Autodesk Inventor part; units mm, degrees
ref_plane "YZ Plane" through (0, 0, 0) normal (1, 0, 0) x (0, 1, 0)
ref_plane "XZ Plane" through (0, 0, 0) normal (0, 1, 0) x (-1, 0, 0)
ref_plane "XY Plane" through (0, 0, 0) normal (0, 0, 1) x (1, 0, 0)
sketch "Sketch1" plane through (0, 0, 0) normal (0, 1, 0) x (-1, 0, 0)
  line L0 (-9.2054, 64.0966) -> (-85.4054, 64.0966)
  line L1 (-85.4054, 64.0966) -> (-85.4054, -88.3034)
  line L2 (-85.4054, -88.3034) -> (-9.2054, -88.3034)
  line L3 (-9.2054, -88.3034) -> (-9.2054, 64.0966)
  point P0 (0, 0)
  dimension "d0" = 152.4
  dimension "d1" = 76.2
extrude "Plate1" add sketch "Sketch1" along normal blind 3.048
sketch "Sketch2" plane through (82.3574, 0, -88.3034) normal (1, 0, 0) x (0, 1, 0)
  line L0 (0, 152.4) -> (0, 0)
  line L1 (0, 0) -> (152.4, 0)
  line L2 (152.4, 0) -> (152.4, 152.4)
  line L3 (152.4, 152.4) -> (0, 152.4)
edge flange "Flange1" height 152.4 angle 90 thickness 3.048 bend radius 3.048 thickness toward (1, 0, 0) relief tear relief width 3.048 relief depth 1.524 edges at (85.4054, 3.048, -12.1034) wall of the first edge with corners at (82.3574, 0, 64.0966) (82.3574, 0, -88.3034) (82.3574, 152.4, -88.3034) (82.3574, 152.4, 64.0966)
bend "Bend1"
corner "Corner1"
sketch "Sketch3" plane through (85.4054, 152.4, 64.0966) normal (1, 0, 0) x (0, 0, -1)
  circle A0 centre (57.15, -76.2) radius 38.1
  line L0 (152.4, 0) -> (152.4, -146.304)
  line L1 (152.4, -152.4) -> (0, -152.4)
  point P0 (64.0966, -152.4)
  dimension "d13" = 76.2
  dimension "d14" = 95.25
  dimension "d15" = 76.2
extrude "Cut1" cut sketch "Sketch3" against normal blind 3.048
sketch "Sketch4" plane through (85.4054, 152.4, 64.0966) normal (1, 0, 0) x (0, 0, -1)
  circle A0 centre (57.15, -76.2) radius 38.1
  line L0 (19.05, -76.2) -> (19.05, 0)
  line L1 (19.05, 0) -> (31.75, 0)
  line L2 (0, 0) -> (152.4, 0)
  line L3 (19.05, 0) -> (31.75, 0)
  line L4 (31.75, 0) -> (31.75, -47.8019)
  arc A1 (31.75, -47.8019) -> (19.05, -76.2) centre (57.15, -76.2) ccw
  point P0 (64.0966, -152.4)
  dimension "d18" = 12.7
extrude "Cut2" cut sketch "Sketch4" against normal blind 3.048 contours A0 L0 L1 L4
sketch "Sketch5" plane through (82.3574, 149.352, 32.3466) normal (0, 1, 0) x (-1, 0, 0)
  line L0 (0, -120.65) -> (0, 0)
  line L1 (0, 0) -> (-114.3, 0)
  line L2 (-114.3, 0) -> (-114.3, -120.65)
  line L3 (-114.3, -120.65) -> (0, -120.65)
edge flange "Flange2" height 114.3 angle 90 thickness 3.048 bend radius 3.048 thickness toward (0, 1, 0) relief tear relief width 3.048 relief depth 1.524 edges at (85.4054, 152.4, -27.9784) wall of the first edge with corners at (82.3574, 149.352, -88.3034) (82.3574, 149.352, 32.3466) (196.6574, 149.352, 32.3466) (196.6574, 149.352, -88.3034)
bend "Bend2"
corner "Corner2"
sketch "Sketch6" plane through (196.6574, 152.4, 32.3466) normal (0, 1, 0) x (1, 0, 0)
  line L0 (0, 120.65) -> (0, 0)
  line L1 (0, 0) -> (-108.204, 0)
  point P0 (-196.6574, 32.3466)
sketch "Sketch7" plane through (82.3574, 149.352, 64.0966) normal (0, 1, 0) x (-1, 0, 0)
  line L0 (0, -19.05) -> (0, 0)
  line L1 (0, 0) -> (-44.45, 0)
  line L2 (-44.45, 0) -> (-44.45, -19.05)
  line L3 (-44.45, -19.05) -> (0, -19.05)
edge flange "Flange3" height 44.45 angle 90 thickness 3.048 bend radius 3.048 thickness toward (0, 1, 0) relief tear relief width 3.048 relief depth 1.524 edges at (85.4054, 152.4, 54.5716) wall of the first edge with corners at (82.3574, 149.352, 45.0466) (82.3574, 149.352, 64.0966) (126.8074, 149.352, 64.0966) (126.8074, 149.352, 45.0466)
bend "Bend3"
corner "Corner3"
sketch "Sketch8" plane through (196.6574, 152.4, 32.3466) normal (0, 1, 0) x (1, 0, 0)
  circle A0 centre (-19.05, 95.25) radius 6.35
  line L0 (0, 120.65) -> (0, 0)
  circle A1 centre (-19.05, 25.4) radius 6.35
  point P0 (-196.6574, 32.3466)
  dimension "d46" = 12.7
  dimension "d47" = 19.05
  dimension "d48" = 69.85
extrude "Cut4" cut sketch "Sketch8" against normal blind 3.048 contours A0
sketch "Sketch9" plane through (126.8074, 152.4, 64.0966) normal (0, 1, 0) x (1, 0, 0)
  circle A0 centre (-19.05, 9.525) radius 4.7625
  line L0 (0, 0) -> (-38.354, 0)
  line L1 (0, 19.05) -> (0, 0)
  point P0 (-126.8074, 64.0966)
  dimension "d51" = 9.525
  dimension "d52" = 9.525
  dimension "d53" = 19.05
extrude "Cut5" cut sketch "Sketch9" against normal blind 3.048
sketch "Sketch10" plane through (196.6574, 152.4, 32.3466) normal (0, 1, 0) x (1, 0, 0)
  circle A0 centre (-19.05, 25.4) radius 6.35
  line L0 (0, 120.65) -> (0, 0)
  circle A1 centre (-19.05, 95.25) radius 6.35
  point P0 (-196.6574, 32.3466)
  dimension "d56" = 12.7
  dimension "d57" = 19.05
  dimension "d58" = 69.85
extrude "Cut6" cut sketch "Sketch10" against normal blind 3.048 contours A0
sketch "Sketch11" plane through (0, 3.048, 0) normal (0, 1, 0) x (1, 0, 0)
  circle A0 centre (28.2554, -54.5716) radius 3.175
  circle A1 centre (66.3554, -54.5716) radius 3.175
  line L0 (79.3094, -64.0966) -> (9.2054, -64.0966)
  line L1 (9.2054, -64.0966) -> (9.2054, 88.3034)
  line L2 (9.2054, 88.3034) -> (79.3094, 88.3034)
  circle A2 centre (28.2554, 78.7784) radius 3.175
  circle A3 centre (66.3554, 81.9534) radius 3.175
  point P0 (0, 0)
  dimension "d61" = 6.35
  dimension "d62" = 6.35
  dimension "d63" = 38.1
  dimension "d64" = 9.525
  dimension "d65" = 9.525
  dimension "d67" = 19.05
  dimension "d68" = 9.525
  dimension "d69" = 6.35
  dimension "d70" = 19.05
  dimension "d71" = 6.35
  dimension "d72" = 6.35
sketch "Sketch12" plane through (0, 3.048, 0) normal (0, 1, 0) x (1, 0, 0)
  circle A0 centre (66.3554, 78.7784) radius 3.175
  line L0 (9.2054, 88.3034) -> (79.3094, 88.3034)
  line L1 (9.2054, -64.0966) -> (9.2054, 88.3034)
  point P0 (0, 0)
  dimension "d73" = 6.35
  dimension "d74" = 9.525
  dimension "d75" = 57.15
extrude "Cut7" cut sketch "Sketch11" against normal blind 3.048 contours A0 | A1 | A2
hole "Hole1" at (66.3554, 3.048, -78.7784) direction (0, -1, 0) diameter 6.35 depth 3.048 tip angle 118
equation "\"d16\" = Thickness"
equation "\"d19\" = Thickness"
equation "\"d49\" = Thickness"
equation "\"d54\" = Thickness"
equation "\"d59\" = Thickness"
equation "\"d76\" = Thickness"
equation "\"d83\" = Thickness"
equation "\"d3\" = BendReliefWidth"
equation "\"d4\" = BendReliefDepth"
equation "\"d5\" = MinimumRemnant"
equation "\"d6\" = BendRadius"
equation "\"d9\" = BendRadius"
equation "\"d10\" = CornerReliefSize"
equation "\"d11\" = GapSize"
equation "\"d12\" = JacobiRadiusSize"
equation "\"d21\" = BendReliefWidth"
equation "\"d22\" = BendReliefDepth"
equation "\"d23\" = MinimumRemnant"
equation "\"d24\" = BendRadius"
equation "\"d27\" = BendRadius"
equation "\"d28\" = CornerReliefSize"
equation "\"d29\" = GapSize"
equation "\"d30\" = JacobiRadiusSize"
equation "\"d34\" = BendReliefWidth"
equation "\"d35\" = BendReliefDepth"
equation "\"d36\" = MinimumRemnant"
equation "\"d37\" = BendRadius"
equation "\"d40\" = BendRadius"
equation "\"d41\" = CornerReliefSize"
equation "\"d42\" = GapSize"
equation "\"d43\" = JacobiRadiusSize"
equation "\"BendRadius\" = Thickness"
equation "\"BendReliefWidth\" = Thickness"
equation "\"BendReliefDepth\" = 0.5 * Thickness"
equation "\"CornerReliefSize\" = 4 * Thickness"
equation "\"MinimumRemnant\" = 2 * Thickness"
equation "\"TransitionRadius\" = BendRadius"
equation "\"JacobiRadiusSize\" = BendRadius"
equation "\"GapSize\" = Thickness"
equation "\"d2\" = BendRadius"
properties part number "Tape Measure Dispenser Side 1"
Check sheet for the modelled part. Datum: model origin and axes. Units: mm. A direction names the side the tool comes from. Round coordinates to 2 decimals unless told otherwise and drop trailing zeros. Loops run counter-clockwise (first coordinate to the right, second up) from the corner with the lowest first, then second, coordinate; pieces in that order, holes last. Notation, with made-up numbers: (13.25, -9.75) -> (28.25, -9.75) arc R20 cw to (28.25, 13.25) -> close; hole circle Ø5 at (-7.75, 85.5). An arc over 180 degrees is marked (long way). Put each result on its own line as item: value. Start each with the question number.
1. Section check C-C (x = 177). Enter the section's corners in (y, z), plus the area to 3 significant figures.
2. Gauge pin test, flat ends, axial feed: pin 1 (0.9 mm diameter, centred on y = 151, z = 59, fed in from +X); pin 2 (21 mm diameter, centred on x = 51.5, z = 17.5, fed in from +Y); pin 3 (5 mm diameter, centred on x = 66.36, z = 54.57, fed in from +Y); pin 4 (21 mm diameter, centred on x = 110, z = 51, fed in from -Y). Record the tip position at first contact, or that the pin passes through.
3. Section check A-A (y = 100). Enter the section's corners in (x, z), plus the area to 3 significant figures.
4. Access from +Z, -Z, +X, -X, +Y, -Y to the whole of each face (thin tool, end or side, straight path). Record for faces 4 (the face through (85.405, 62, -30)), 5 (the face through (112.2, 152.4, 56.8)), 6 (the face through (123, 150, 32.347)), 7 (the face through (104.25, 150.9, 51.35)), 8 (the face through (45, 3.048, -11)).
5. Scan lines: probe 1 along Y at (x, z) = (186, 22.5); probe 2 along Y at (x, z) = (57, 54.5); probe 3 along X at (y, z) = (13, 22). Record each from-to range of solid material in increasing order.
6. Section check D-D (y = 52.5). Enter the section's corners in (x, z), plus the area to 3 significant figures.
7. Draft check along Z on faces 1 (the face through (85, 126, 45.047)), 2 (the face through (25.915, 1.545, -80.924)), 3 (the face through (142, 149.352, -27)). Enter one of: +Z half, -Z half, draft (parallel to the pull), parting line (faces both ways), or undercut.
8. Section check B-B (z = 16.5). Enter the section's corners in (x, y).
Findings:
1. outline: (149.35, -88.3) -> (152.4, -88.3) -> (152.4, -69.22) -> (149.35, -69.22) -> close; (149.35, -56.58) -> (152.4, -56.58) -> (152.4, 0.63) -> (149.35, 0.63) -> close; (149.35, 13.27) -> (152.4, 13.27) -> (152.4, 32.35) -> (149.35, 32.35) -> close
1. area: 291 mm^2
2. pin 1: stops at x = 126.81
2. pin 2: stops at y = 3.05
2. pin 3: passes through
2. pin 4: stops at y = 149.35
3. outline: (82.36, -88.3) -> (85.41, -88.3) -> (85.41, -22.81) -> (82.36, -22.81) -> close; (82.36, 45.05) -> (85.41, 45.05) -> (85.41, 64.1) -> (82.36, 64.1) -> close
3. area: 258 mm^2
4. face 4: +Z, -Z, +X, -Y
4. face 5: +Z, -Z, +X, -X, +Y
4. face 6: +X, -X, +Y
4. face 7: +Y, -Y
4. face 8: +Z, -Z, -X, +Y
5. probe 1: y = 149.35 to 152.4
5. probe 2: y = 0 to 3.05
5. probe 3: x = 82.36 to 85.41
6. outline: (82.36, -88.3) -> (85.41, -88.3) -> (85.41, -22.88) -> (82.36, -22.88) -> close; (82.36, 36.78) -> (85.41, 36.78) -> (85.41, 64.1) -> (82.36, 64.1) -> close
6. area: 283 mm^2
7. face 1: undercut
7. face 2: undercut
7. face 3: draft
8. outline: (9.21, 0) -> (79.31, 0) arc R6.1 ccw to (85.41, 6.1) -> (85.41, 39.32) -> (82.36, 39.32) -> (82.36, 6.1) arc R3.05 cw to (79.31, 3.05) -> (9.21, 3.05) -> close; (82.36, 113.08) -> (85.41, 113.08) -> (85.41, 146.3) arc R3.05 cw to (88.45, 149.35) -> (196.66, 149.35) -> (196.66, 152.4) -> (88.45, 152.4) arc R6.1 ccw to (82.36, 146.3) -> close
